Source: CAD feature listing. Evaluate the final solid. Frame: model axes, mm. Face numbers are marked on the shaded views. A direction names the side the tool comes from. Give positions to 0.01 mm unless a question says otherwise; leave off trailing zeros. Order: outer loops, then holes, each group sorted by start corner. A loop starts at its lowest first (then second) coordinate and runs counter-clockwise, first axis right, second up. Notation, with made-up numbers: (-39.5, 45.5) -> (-18.5, 45.5) arc R18 ccw to (-18.5, 62.5) -> close; hole circle Ø9 at (9.25, -27.75). An arc over 180 degrees is marked (long way). Use one line per item in the form item = value. Start each with the question number.
from build123d import *

# Parameters (mm, degrees)
F1_DEPTH = 19.05


with BuildPart() as f1:
    # F0 (on Front) → F1 (new body)
    with BuildSketch(Plane.XZ):
        with BuildLine():
            Line((-15.875, 0), (0, 0))
            Line((0, 0), (15.875, 0))
            Line((15.875, 0), (15.875, 44.45))
            Line((15.875, 44.45), (25.4, 44.45))
            Line((25.4, 44.45), (25.4, 48.797853))
            ThreePointArc((25.4, 48.797853), (25.106103, 50.707335), (24.251615, 52.440063))
            Line((24.251615, 52.440063), (11.733902, 70.31721))
            ThreePointArc((11.733902, 70.31721), (9.46439, 72.307519), (6.532287, 73.025))
            Line((6.532287, 73.025), (0, 73.025))
            Line((0, 73.025), (-6.532287, 73.025))
            ThreePointArc((-6.532287, 73.025), (-9.46439, 72.307519), (-11.733902, 70.31721))
            Line((-11.733902, 70.31721), (-24.251615, 52.440063))
            ThreePointArc((-24.251615, 52.440063), (-25.106103, 50.707335), (-25.4, 48.797853))
            Line((-25.4, 48.797853), (-25.4, 44.45))
            Line((-25.4, 44.45), (-15.875, 44.45))
            Line((-15.875, 44.45), (-15.875, 0))
        make_face()
    extrude(amount=F1_DEPTH)


solid = f1.part
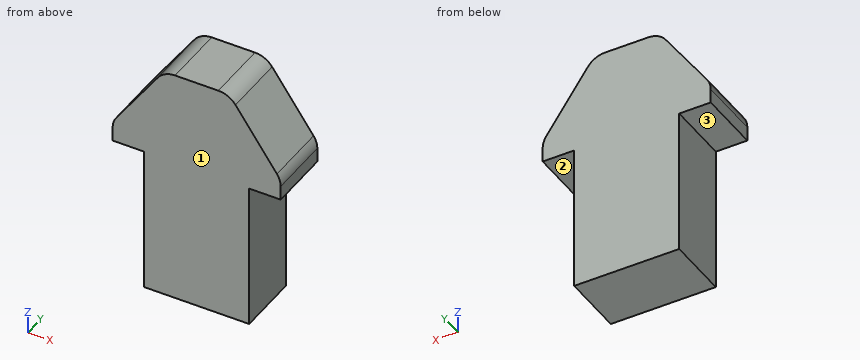
1) Cut plane B-B, the plane z = 36. Return the cut outline in (x, y) (3 decimals), plus the area to 3 significant figures.
2) Pin query (flat end, axial travel): pin 1 (5.5 mm diameter, centred on y = -10.5, z = 20, fed in from -X) (3 decimals); pin 2 (8 mm diameter, centred on x = -13.5, y = -14, fed in from +Z); pin 3 (5 mm diameter, centred on x = -18.5, y = -5, fed in from -Z). Return the tip coordinate at first contact, or that it passes through.
3) Cut plane C-C, the plane x = 21. Return the cut outline in (y, z).
4) Material intervals for probe 1 along X at (y, z) = (-14.75, 42) (3 decimals); probe 2 along Z at (x, y) = (11.5, -2); probe 3 along Z at (x, y) = (-7, -6.25), sorted ascending.
5) Reachability of the marked faces 1, 2 and 3 from +Z, -Z, +X, -X, +Y, -Y: full face, straight path, thin tool, end or side. Return the list, or none.
6) Cut plane A-A, the plane y = -11.5. Return the cut outline in (x, z) (3 decimals).
Output values:
q1.outline = (-15.875, -19.05) -> (15.875, -19.05) -> (15.875, 0) -> (-15.875, 0) -> close
q1.area = 605 mm^2
q2.pin_1 = -15.875
q2.pin_2 = 72.29
q2.pin_3 = 44.45
q3.outline = (-19.05, 44.45) -> (0, 44.45) -> (0, 57.08) -> (-19.05, 57.08) -> close
q4.probe_1 = -15.875 to 15.875
q4.probe_2 = 0 to 70.63
q4.probe_3 = 0 to 73.01
q5.face_1 = +Z, -Z, +X, -X, -Y
q5.face_2 = -Z, +X, +Y, -Y
q5.face_3 = -Z, -X, +Y, -Y
q6.outline = (-25.4, 44.45) -> (-15.875, 44.45) -> (-15.875, 0) -> (15.875, 0) -> (15.875, 44.45) -> (25.4, 44.45) -> (25.4, 48.798) arc R6.35 ccw to (24.252, 52.44) -> (11.734, 70.317) arc R6.35 ccw to (6.532, 73.025) -> (-6.532, 73.025) arc R6.35 ccw to (-11.734, 70.317) -> (-24.252, 52.44) arc R6.35 ccw to (-25.4, 48.798) -> close
